Verification items for the finished model (mm, model axes). Coordinates: 2 decimals unless noted, no trailing zeros. Loops run counter-clockwise (first coordinate to the right, second up) from the corner with the lowest first, then second, coordinate; pieces in that order, holes last. Notation, with made-up numbers: (22, 80) - (80, 80) arc R32 cw to (80, 117) - close; hole circle Ø3 at (38.5, 28.5). An arc over 180 degrees is marked (long way). Answer as CSV lines item,"result". Start each with the question number.
1. Cross-section at D-D (x = 19). Enter the section's corners in (y, z).
2. Cross-section at A-A (x = 32.48). Enter the section's corners in (y, z).
3. Material ranges on line 1 (Y direction, x = 3.3, z = 15.05) (3 decimals); line 2 (Z direction, x = 7, y = 18.25), recorded low to high. Write a range as [from, to].
4. Cross-section at C-C (y = 3.3). Enter the section's corners in (x, z) (3 decimals).
5. Cross-section at B-B (y = 12.16). Enter the section's corners in (x, z).
6. Gauge pin test, flat ends, axial feed: P1, Ø5, axis at x = 13.5, z = 10.5, coming from the -Y side; P2, Ø9.5, axis at x = 10, y = 11.5, coming from the -Z side; P3, Ø1.5, axis at y = 12.5, z = -3, coming from the +X side. Record the tip position at first contact, or that the pin passes through.
```python
from build123d import *

# Parameters (mm, degrees)
SKIZZE1_W                       = 34.48
SKIZZE1_H                       = 19.24
AUFSATZ_LINEAR_AUSTRAGEN1_DEPTH = 15.24
SKIZZE2_R                       = 0.375
SCHNITT_LINEAR_AUSTRAGEN1_DEPTH = 0.3
SKIZZE3_R                       = 0.4
AUFSATZ_LINEAR_AUSTRAGEN2_DEPTH = 5


with BuildPart() as part:
    # Skizze1 → Aufsatz-Linear austragen1 (new body)
    with BuildSketch(Plane.XY):
        with Locations((17.24, 9.62)):
            Rectangle(SKIZZE1_W, SKIZZE1_H)
    extrude(amount=AUFSATZ_LINEAR_AUSTRAGEN1_DEPTH)

    # Skizze2 → Schnitt-Linear austragen1 (cut)
    with BuildSketch(Plane.XY.offset(15.24)):
        with Locations((3.3, 3.3)):
            Circle(SKIZZE2_R)
    extrude(amount=-SCHNITT_LINEAR_AUSTRAGEN1_DEPTH, mode=Mode.SUBTRACT)

    # Skizze3 → Aufsatz-Linear austragen2 (add)
    with BuildSketch(Plane(origin=(0, 0, 0), x_dir=(-1, 0, 0), z_dir=(0, 0, -1))):
        with Locations((-32.48, 17.24)):
            Circle(SKIZZE3_R)
        with Locations((-32.48, 2)):
            Circle(SKIZZE3_R)
        with Locations((-2, 12.16)):
            Circle(SKIZZE3_R)
        with Locations((-2, 7.08)):
            Circle(SKIZZE3_R)
    extrude(amount=AUFSATZ_LINEAR_AUSTRAGEN2_DEPTH)


solid = part.part
```
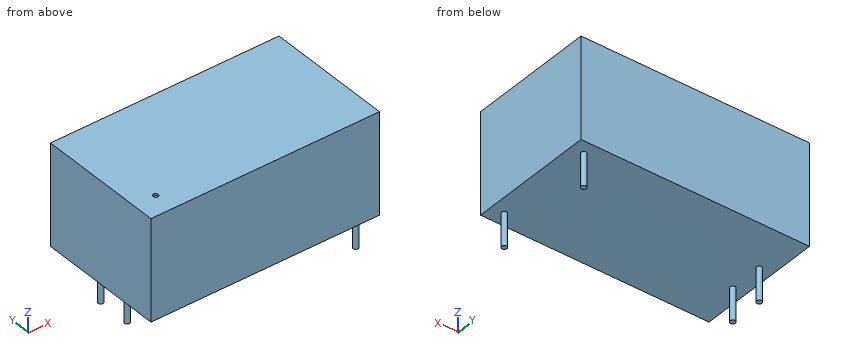
Values follow:
1,outline,"(0, 0) - (19.24, 0) - (19.24, 15.24) - (0, 15.24) - close"
2,outline,"(0, 0) - (1.6, 0) - (1.6, -5) - (2.4, -5) - (2.4, 0) - (16.84, 0) - (16.84, -5) - (17.64, -5) - (17.64, 0) - (19.24, 0) - (19.24, 15.24) - (0, 15.24) - close"
3,line 1,"y = [0, 2.925], [3.675, 19.24]"
3,line 2,"z = [0, 15.24]"
4,outline,"(0, 0) - (34.48, 0) - (34.48, 15.24) - (3.675, 15.24) - (3.675, 14.94) - (2.925, 14.94) - (2.925, 15.24) - (0, 15.24) - close"
5,outline,"(0, 0) - (1.6, 0) - (1.6, -5) - (2.4, -5) - (2.4, 0) - (34.48, 0) - (34.48, 15.24) - (0, 15.24) - close"
6,P1,"stops at y = 0"
6,P2,"stops at z = 0"
6,P3,"stops at x = 2.4"
